Design review of the part built by this model. Coordinates are the model's own, in mm. Face numbers are marked on the shaded views. A direction names the side the tool comes from. Coordinates: 2 decimals unless noted, no trailing zeros. Order: outer loops, then holes, each group sorted by start corner. A loop starts at its lowest first (then second) coordinate and runs counter-clockwise, first axis right, second up. Notation, with made-up numbers: M 52,42 L 63,42 A9 ccw 63,53 Z; hole C 10,-1 d1. An arc over 180 degrees is marked long. Answer as a JSON object with one key per item and string values.
from build123d import *

# Parameters (mm, degrees)
MAIN_BODY_PROFILE_R     = 11.1125
MAIN_BODY_EXTRUDE_DEPTH = 28.575
HEXAGON_BODY_DEPTH      = 12.7
TIP_PROFILE_R           = 8.9281
TIP_BODY_DEPTH          = 6.35
BACK_POWDER_HOLE_D      = 12.7
BACK_POWDER_HOLE_DEPTH  = 31.109535069
BACK_POWDER_HOLE_TIP    = 3.815464931
SCREW_HOLES_AT_2_COUNT  = 2
SCREW_HOLES_AT_2_PITCH  = 6.985
SKETCH12_R              = 2.8575
THROUGH_HOLES_DEPTH     = 41.246641376


with BuildPart() as part:
    # Main Body Profile → Main Body Extrude (new body)
    with BuildSketch(Plane(origin=(0, 0, 0), x_dir=(1, 0, 0), z_dir=(0, 1, 0))):
        Circle(MAIN_BODY_PROFILE_R)
    extrude(amount=MAIN_BODY_EXTRUDE_DEPTH)

    # Hexagon Profile → Hexagon Body (add)
    with BuildSketch(Plane(origin=(0, 28.575, 0), x_dir=(1, 0, 0), z_dir=(0, 1, 0))):
        Polygon((5.499261314, 9.525), (-5.499261314, 9.525), (-10.998522628, 0), (-5.499261314, -9.525), (5.499261314, -9.525), (10.998522628, 0), align=None)
    extrude(amount=HEXAGON_BODY_DEPTH)

    # Tip Profile → Tip Body (add)
    with BuildSketch(Plane.XZ):
        Circle(TIP_PROFILE_R)
    extrude(amount=TIP_BODY_DEPTH)

    # Back Powder Hole
    with Locations(Plane(origin=(0, -6.35, 0), x_dir=(-1, 0, 0), z_dir=(0, -1, 0))):
        with Locations((0, 0)):
            Hole(BACK_POWDER_HOLE_D / 2, depth=BACK_POWDER_HOLE_DEPTH)
            with Locations((0, 0, -(BACK_POWDER_HOLE_DEPTH + BACK_POWDER_HOLE_TIP / 2))):  # 118° drill point
                Cone(0, BACK_POWDER_HOLE_D / 2, BACK_POWDER_HOLE_TIP, mode=Mode.SUBTRACT)

    # Sketch11 → Screw Holes (revolve, cut)
    with BuildSketch(Plane(origin=(0, 33.896641376, 3.4925), x_dir=(0, 0, -1), z_dir=(1, 0, 0))):
        Polygon((0, 0), (0, 7.378358624), (1.63195, 7.378358624), (1.63195, 1.028358553), (2.8575, 0), align=None)
    screw_holes = revolve(axis=Axis((0, 27.546641376, 3.4925), (0, 1, 0)), mode=Mode.SUBTRACT)

    # Screw Holes at 2: Screw Holes ×2
    with Locations(*[(0, 0, -i * SCREW_HOLES_AT_2_PITCH) for i in range(1, SCREW_HOLES_AT_2_COUNT)]):
        add(screw_holes, mode=Mode.SUBTRACT)

    # Sketch12 → Through Holes (cut, through all)
    with BuildSketch(Plane(origin=(0, 33.896641376, 0), x_dir=(1, 0, 0), z_dir=(0, 1, 0))):
        with Locations((0, 3.4925)):
            Circle(SKETCH12_R)
        with Locations((0, -3.4925)):
            Circle(SKETCH12_R)
    extrude(amount=-THROUGH_HOLES_DEPTH, mode=Mode.SUBTRACT)

    # Sketch13 → Revolved Cut (revolve, cut)
    with BuildSketch(Plane.XY):
        Polygon((-8.9281, 0), (-7.696200006, 0), (-8.9281, -0.7112378), align=None)
    revolve(axis=Axis((0, 0, 0), (0, -1, 0)), mode=Mode.SUBTRACT)


solid = part.part
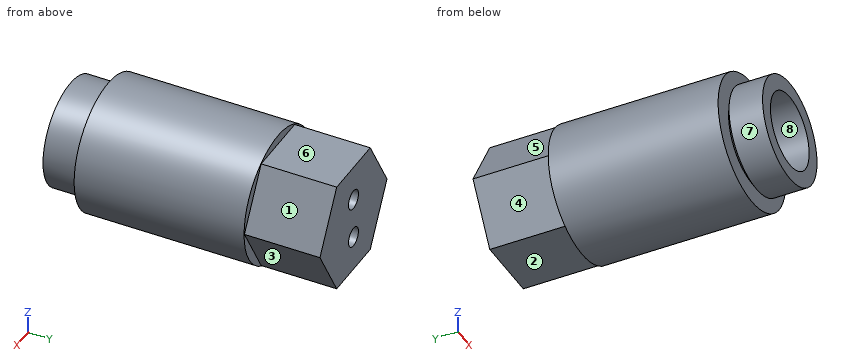
1) Tool access review of the marked faces 1, 2, 3, 4 and 5: name each direction out of +Z, -Z, +X, -X, +Y, -Y from which nothing blocks a thin tool from reaching the whole face with its end or side.
Taken from the geometry:
{"face 1": "+Z, +X, +Y", "face 2": "-Z, +X, -X, +Y", "face 3": "-Z, +X, +Y", "face 4": "-Z, -X, +Y", "face 5": "+Z, -X, +Y"}
2) Mouldability with a two-part tool opening along Z and no side actions: class the marked faces 6, 7 and 8 as released by +Z, released by -Z, zero draft, split by the parting line, or undercut.
Taken from the geometry:
{"face 6": "released by +Z", "face 7": "split by the parting line", "face 8": "undercut"}
3) Add section A-A (y = 30.5). State the section outline as (x, z) points (1 decimal).
Taken from the geometry:
{"outline": "M -11,0 L -5.5,-9.5 L 5.5,-9.5 L 11,0 L 5.5,9.5 L -5.5,9.5 Z; hole C 0,-3.5 d5.7; hole C 0,3.5 d5.7"}
4) To check wall thickness, follow L1, parallel to Z at x = 0, y = 37.5 (3 decimals); L2, parallel to Z at x = 0, y = 27.25; L3, parallel to Y at x = -7.5, z = -7 (3 decimals). State the ranges of each line that lie inside material, in increasing order.
Taken from the geometry:
{"L1": "z = -9.525 to -5.124, -1.861 to 1.861, 5.124 to 9.525", "L2": "z = -11.11 to -6.35, 6.35 to 11.11", "L3": "y = 0 to 28.575"}
5) Insertion check: pin 1 Ø4.5 at (x, z) = (0, 3.49) entering from -Y; pin 2 Ø1.5 at (y, z) = (10.5, 2.5) entering from +X; pin 3 Ø5.5 at (x, y) = (0, 33) entering from +Z (3 decimals); pin 4 Ø2.5 at (x, z) = (0, 3.49) entering from +Y. Each pin has a flat end and moves straight along its axis. Give the tip position at first contact, or say it passes through.
Taken from the geometry:
{"pin 1": "stops at y = 34.4", "pin 2": "stops at x = 10.97", "pin 3": "stops at z = 9.525", "pin 4": "passes through"}
